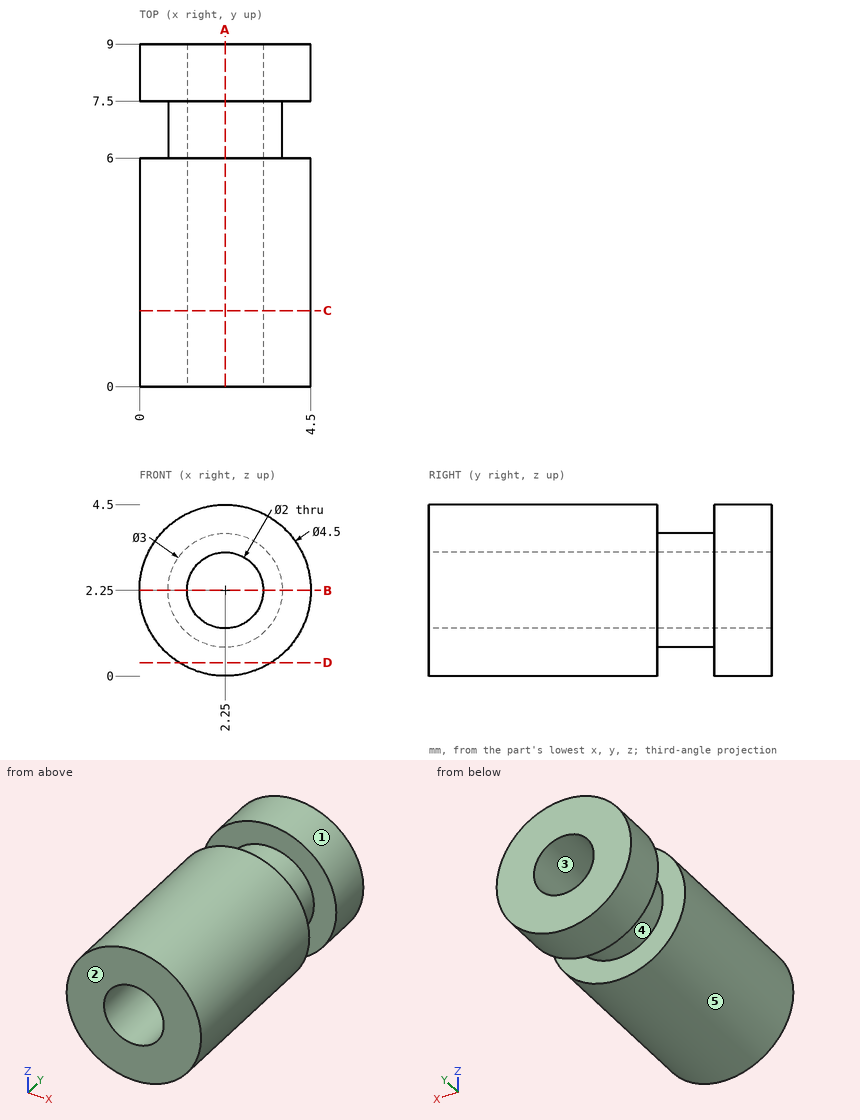
Job drawing, mm, ordinate dimensions from the low corner. One solid piece. A direction names the side the tool comes from. Give positions to 0.01 mm unless a question says otherwise; leave off trailing zeros. Order: outer loops, then holes, each group sorted by start corner. A loop starts at its lowest first (then second) coordinate and runs counter-clockwise, first axis right, second up. Notation, with made-up numbers: (2.25, 48.25) -> (38.25, 48.25) arc R9 cw to (38.25, 52.25) -> close; hole circle Ø7 at (83, 51). An arc over 180 degrees is marked (long way). Return JSON: item names as keys, results as strings.
Q1. Flat gauge pins, fed straight in: pin 1 (2 mm diameter, centred on x = 1, y = 3, fed in from -Z); pin 2 (2 mm diameter, centred on x = 0.5, y = 2.5, fed in from +Z). Where does each tip first touch, or does it go through?
Working result:
{"pin 1": "z = 0.01", "pin 2": "z = 4.37"}
Q2. Saw through at D-D (z = 0.35). Write the cut outline in (x, y), then the cut area to 3 significant figures.
Working result:
{"outline": "(1.04, 0) -> (3.46, 0) -> (3.46, 6) -> (1.04, 6) -> close; (1.04, 7.5) -> (3.46, 7.5) -> (3.46, 9) -> (1.04, 9) -> close", "area": "18.1 mm²"}
Q3. Drill centre lines: line 1 (Y direction, x = 0.95, z = 3.9); line 2 (Z direction, x = 2.25, y = 3.5). Where is each one in solid material? Low to high.
Working result:
{"line 1": "0 to 6, 7.5 to 9", "line 2": "0 to 1.25, 3.25 to 4.5"}
Q4. Saw through at C-C (y = 2). Write the cut outline in (x, z), then the cut area to 3 significant figures.
Working result:
{"outline": "circle Ø4.5 at (2.25, 2.25); hole circle Ø2 at (2.25, 2.25)", "area": "12.8 mm²"}
Q5. Saw through at A-A (x = 2.25). Write the cut outline in (y, z), then the cut area to 4 significant figures.
Working result:
{"outline": "(0, 0) -> (6, 0) -> (6, 0.75) -> (7.5, 0.75) -> (7.5, 0) -> (9, 0) -> (9, 1.25) -> (0, 1.25) -> close; (0, 3.25) -> (9, 3.25) -> (9, 4.5) -> (7.5, 4.5) -> (7.5, 3.75) -> (6, 3.75) -> (6, 4.5) -> (0, 4.5) -> close", "area": "20.25 mm²"}
Q6. Which spindle directions (+Z, -Z, +X, -X, +Y, -Y) get a long thin tool onto all of the face, cutting with end or side? Do the marked faces 4 and 5. Say none if no direction does.
Working result:
{"face 4": "none", "face 5": "+Y, -Y"}
Q7. Mould opens along X. For the marked faces 1, 2 and 3 say: pulls with the +X half, pulls with the -X half, needs draft (parallel to the pull), parting line crosses it, or undercut.
Working result:
{"face 1": "parting line crosses it", "face 2": "needs draft", "face 3": "undercut"}
Q8. Saw through at B-B (z = 2.25). Write the cut outline in (x, y), then the cut area to 4 significant figures.
Working result:
{"outline": "(0, 0) -> (1.25, 0) -> (1.25, 9) -> (0, 9) -> (0, 7.5) -> (0.75, 7.5) -> (0.75, 6) -> (0, 6) -> close; (3.25, 0) -> (4.5, 0) -> (4.5, 6) -> (3.75, 6) -> (3.75, 7.5) -> (4.5, 7.5) -> (4.5, 9) -> (3.25, 9) -> close", "area": "20.25 mm²"}
